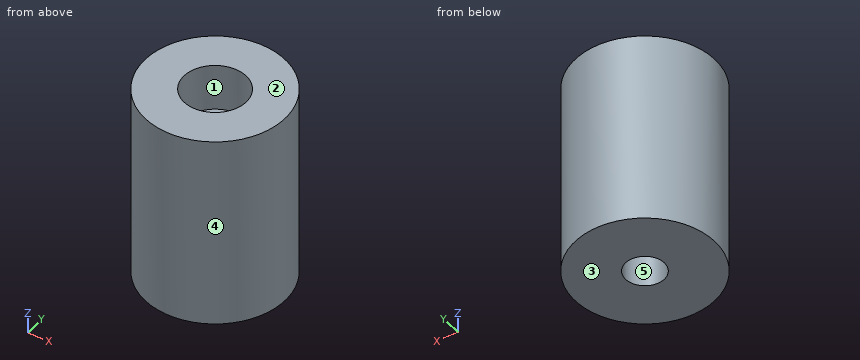
```python
from build123d import *

# Parameters (mm, degrees)
SKETCH045_R              = 9
PAD027_DEPTH             = 25
SKETCH046_R              = 2.5
POCKET021_DEPTH          = 6
SKETCH047_R              = 4
POCKET022_DEPTH          = 6
CLONE040_PLACEMENT_ANGLE = 180


with BuildPart() as part:
    # Sketch045 → Pad027 (new body)
    with BuildSketch(Plane.XY):
        Circle(SKETCH045_R)
    extrude(amount=PAD027_DEPTH)

    # Sketch046 (on Face3 of Pad027) → Pocket021 (cut)
    with BuildSketch(Plane.XY.offset(25)):
        Circle(SKETCH046_R)
    extrude(amount=-POCKET021_DEPTH, mode=Mode.SUBTRACT)

    # Sketch047 (on Face2 of Pocket021) → Pocket022 (cut)
    with BuildSketch(Plane(origin=(0, 0, 0), x_dir=(1, 0, 0), z_dir=(0, 0, -1))):
        Circle(SKETCH047_R)
    extrude(amount=-POCKET022_DEPTH, mode=Mode.SUBTRACT)


with BuildPart() as part_1:
    # Clone040 placement: moved
    add(part.part.moved(Location((-310, -25, 82))).rotate(Axis((-310, -25, 82), (0, 1, 0)), CLONE040_PLACEMENT_ANGLE))


solid = part_1.part
```
Part model, mm, in its own coordinate system. Face numbers are marked on the shaded views. A direction names the side the tool comes from. Round coordinates to 2 decimals unless told otherwise and drop trailing zeros. Order: outer loops, then holes, each group sorted by start corner. A loop starts at its lowest first (then second) coordinate and runs counter-clockwise, first axis right, second up. Notation, with made-up numbers: M 26,7.5 L 71,7.5 A21 cw 71,21.5 Z; hole C 5.25,18.25 d9. An arc over 180 degrees is marked long. Put each result on its own line as item: value. Start each with the question number.
1. Two-plate mould, pull along Y, no slides. Class the marked faces 3, 4 and 5: +Y half, -Y half, draft (parallel to the pull), parting line (faces both ways), or undercut.
2. Slice it at A-A on y = -25. List the corners of the cut face in (x, z), then the cut area to 3 significant figures.
3. Tool access for the marked faces 1 and 2: list every direction of +Z, -Z, +X, -X, +Y, -Y with a clear straight run to the whole face (end or side of a thin tool).
4. Slice it at D-D on x = -304.5. List the corners of the cut face in (y, z).
5. Slice it at B-B on x = -310. List the corners of the cut face in (y, z), then the cut area to 3 significant figures.
6. Drill centre lines: probe 1 along Y at (x, z) = (-310, 61.3); probe 2 along Y at (x, z) = (-310, 77.5); probe 3 along Z at (x, y) = (-309, -21.5). Where is each one in solid material? Low to high. Write a range as [from, to].
7. Slice it at C-C on z = 71.25. List the corners of the cut face in (x, y).
8. Drop flat-ended pins along their axis: pin 1 (5 mm diameter, centred on x = -307, y = -25, fed in from +Z); pin 2 (7 mm diameter, centred on x = -310, y = -25, fed in from +Z); pin 3 (5 mm diameter, centred on y = -31, z = 66, fed in from -X); pin 4 (1.5 mm diameter, centred on x = -312.5, z = 77, fed in from +Y). Give the stop position or say it passes through.
Findings:
1. face 3: draft
1. face 4: parting line
1. face 5: undercut
2. outline: M -319,57 L -312.5,57 L -312.5,63 L -307.5,63 L -307.5,57 L -301,57 L -301,82 L -306,82 L -306,76 L -314,76 L -314,82 L -319,82 Z
2. area: 372 mm2
3. face 1: +Z
3. face 2: +Z, +X, -X, +Y, -Y
4. outline: M -32.12,57 L -17.88,57 L -17.88,82 L -32.12,82 Z
5. outline: M -34,57 L -27.5,57 L -27.5,63 L -22.5,63 L -22.5,57 L -16,57 L -16,82 L -21,82 L -21,76 L -29,76 L -29,82 L -34,82 Z
5. area: 372 mm2
6. probe 1: [-34, -27.5], [-22.5, -16]
6. probe 2: [-34, -29], [-21, -16]
6. probe 3: [57, 76]
7. outline: C -310,-25 d18
8. pin 1: z = 82
8. pin 2: z = 76
8. pin 3: x = -318.29
8. pin 4: y = -16.17
